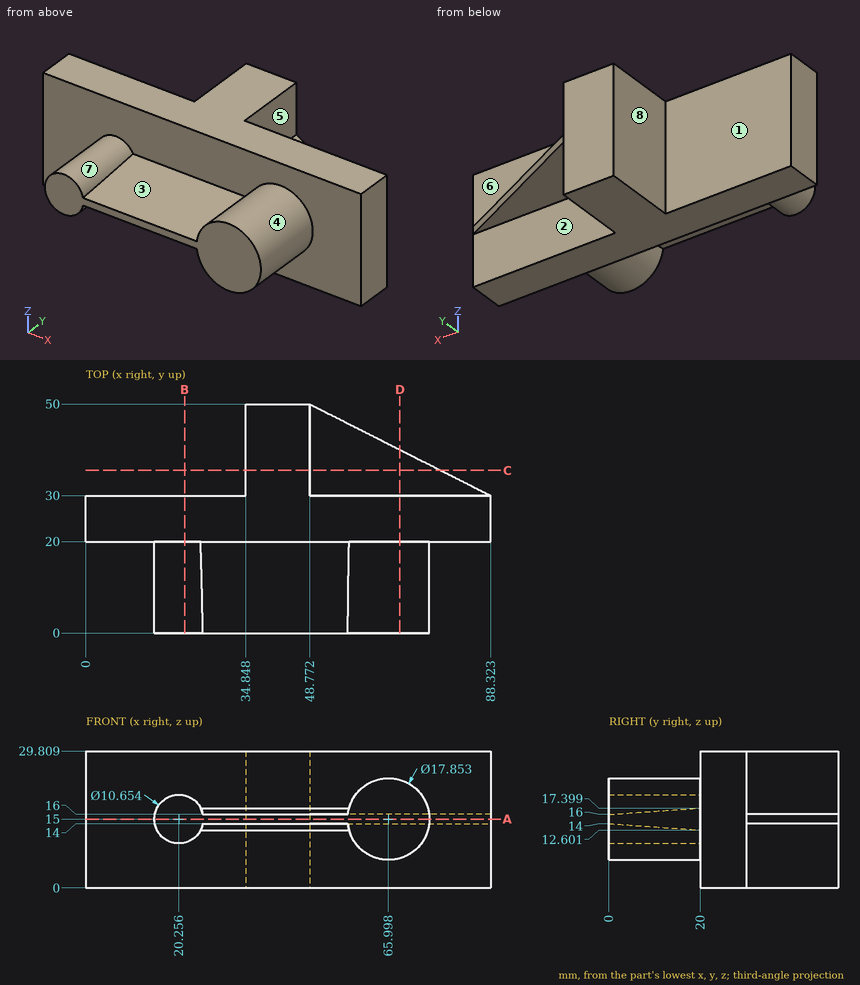
Design review of the part shown in the three views and the two pictorial views. Dimensions are in mm from the part's minimum x, y and z. A direction names the side the tool comes from. Round coordinates to 2 decimals unless told otherwise and drop trailing zeros. Loops run counter-clockwise (first coordinate to the right, second up) from the corner with the lowest first, then second, coordinate; pieces in that order, holes last. Notation, with made-up numbers: (-9.5, 27.25) -> (49.5, 27.25) arc R14 ccw to (49.5, 44.25) -> close; hole circle Ø6 at (33.5, 49). An arc over 180 degrees is marked (long way). Return JSON: item names as keys, results as strings.
(1) Add section A-A on z = 15. Write out the cut boundary in (x, y) (1 decimal), plus the area to 3 significant figures.
Solved:
{"outline": "(0, 20) -> (14.9, 20) -> (14.9, 0) -> (74.9, 0) -> (74.9, 20) -> (88.3, 20) -> (88.3, 30) -> (48.8, 50) -> (34.8, 50) -> (34.8, 30) -> (0, 30) -> close", "area": "2,760 mm2"}
(2) For the marked faces 1, 2, 3 and 4, list the 3-axis set-ups (+Z, -Z, +X, -X, +Y, -Y) from which the entire face can be reached by the end or side of a thin tool; tool diameter is ignored.
Solved:
{"face 1": "+Z, -Z, -X, +Y", "face 2": "-Z, +X, +Y", "face 3": "+Z, -Y", "face 4": "-Y"}
(3) Add section C-C on y = 35.5. Write out the cut boundary in (x, z).
Solved:
{"outline": "(34.85, 0) -> (48.77, 0) -> (48.77, 14) -> (77.45, 14) -> (77.45, 16) -> (48.77, 16) -> (48.77, 29.81) -> (34.85, 29.81) -> close"}
(4) For line 1 (Y direction, x = 61.5, z = 27.75); line 2 (Y direction, x = 48.5, z = 10); line 3 (X direction, y = 42, z = 11.5), list the stretches that pass through material, from the lowest coordinate up.
Solved:
{"line 1": "20 to 30", "line 2": "20 to 50", "line 3": "34.85 to 48.77"}
(5) Add section D-D on x = 68.5. Write out the cut boundary in (y, z).
Solved:
{"outline": "(0, 6.43) -> (20, 6.43) -> (20, 0) -> (30, 0) -> (30, 14) -> (40.02, 14) -> (40.02, 16) -> (30, 16) -> (30, 29.81) -> (20, 29.81) -> (20, 23.57) -> (0, 23.57) -> close"}
(6) Add section B-B on x = 21.5. Write out the cut boundary in (y, z), plus the area to 3 significant figures.
Solved:
{"outline": "(0, 9.82) -> (20, 9.82) -> (20, 0) -> (30, 0) -> (30, 29.81) -> (20, 29.81) -> (20, 20.18) -> (0, 20.18) -> close", "area": "505 mm2"}
(7) The part is to be moulded in two halves that separate along X. For the marked faces 5, 6, 7 and 8, say which applies: released by +X, released by -X, zero draft, split by the parting line, or undercut.
Solved:
{"face 5": "released by +X", "face 6": "zero draft", "face 7": "undercut", "face 8": "released by -X"}
(8) For pin 1 (6 mm diameter, centred on x = 74, z = 4.5, fed in from -Y); pin 2 (5 mm diameter, centred on y = 37, z = 9, fed in from +X); pin 3 (6 mm diameter, centred on x = 71, y = 40.5, fed in from -Z), all flat-tipped, find the tip position at first contact; note any pin that passes through.
Solved:
{"pin 1": "y = 20", "pin 2": "x = 48.77", "pin 3": "z = 14"}
